The listing builds one solid part. Answer for the finished solid, in the listing's coordinates (mm). Give positions to 0.01 mm unless a question says otherwise; leave off trailing zeros. Loops run counter-clockwise (first coordinate to the right, second up) from the corner with the lowest first, then second, coordinate; pieces in that order, holes last. Notation, with made-up numbers: (78.25, 55) - (92.25, 55) arc R23 cw to (92.25, 90) - close; hole circle Ø10 at (1, 35.25). An arc over 180 degrees is marked (long way). Answer in a Markdown table with one row per item. Add a question column.
```python
from build123d import *

# Parameters (mm, degrees)
SKETCH1_R           = 4.25
SKETCH1_R_2         = 1.5
SKETCH1_W           = 40
SKETCH1_H           = 20
BOSS_EXTRUDE1_DEPTH = 6.1
SKETCH2_R           = 10.35
CUT_EXTRUDE1_DEPTH  = 2.55
SKETCH3_R           = 0.75
CUT_EXTRUDE3_DEPTH  = 3.55
CUT_EXTRUDE4_DEPTH  = 6.1


with BuildPart() as part:
    # Sketch1 → Boss-Extrude1 (new body)
    with BuildSketch(Plane(origin=(0, 0, 0), x_dir=(1, 0, 0), z_dir=(0, 1, 0))):
        with BuildLine():
            Line((150, 20), (159.5, 20))
            Line((159.5, 20), (166.5, 20))
            ThreePointArc((166.5, 20), (186.5, 0), (166.5, -20))
            Line((166.5, -20), (159.5, -20))
            Line((159.5, -20), (150, -20))
            Line((150, -20), (0, -20))
            ThreePointArc((0, -20), (-20, 0), (0, 20))
            Line((0, 20), (150, 20))
        make_face()
        with Locations(Location((0, 0, 0), (0, 0, 270))):
            Circle(SKETCH1_R, mode=Mode.SUBTRACT)
        with Locations(Location((165, 4.825, 0), (0, 0, 270))):
            Circle(SKETCH1_R_2, mode=Mode.SUBTRACT)
        with Locations(Location((165, -4.825, 0), (0, 0, 270))):
            Circle(SKETCH1_R_2, mode=Mode.SUBTRACT)
        with Locations(Location((114, 4.825, 0), (0, 0, 270))):
            Circle(SKETCH1_R_2, mode=Mode.SUBTRACT)
        with Locations(Location((114, -4.825, 0), (0, 0, 270))):
            Circle(SKETCH1_R_2, mode=Mode.SUBTRACT)
        with Locations((139.5, 0)):
            Rectangle(SKETCH1_W, SKETCH1_H, mode=Mode.SUBTRACT)
    extrude(amount=BOSS_EXTRUDE1_DEPTH)

    # Sketch2 → Cut-Extrude1 (cut)
    with BuildSketch(Plane(origin=(0, 6.1, 0), x_dir=(1, 0, 0), z_dir=(0, 1, 0))):
        with Locations(Location((0, 0, 0), (0, 0, 270))):
            Circle(SKETCH2_R)
    extrude(amount=-CUT_EXTRUDE1_DEPTH, mode=Mode.SUBTRACT)

    # Sketch3 → Cut-Extrude3 (cut)
    with BuildSketch(Plane(origin=(0, 3.55, 0), x_dir=(1, 0, 0), z_dir=(0, 1, 0))):
        with Locations(Location((-7.52500865, 2.715556079, 0), (0, 0, 270))):
            Circle(SKETCH3_R)
        with Locations(Location((7.52500865, -2.715556079, 0), (0, 0, 270))):
            Circle(SKETCH3_R)
        with Locations(Location((2.715556079, 7.52500865, 0), (0, 0, 270))):
            Circle(SKETCH3_R)
        with Locations(Location((-2.715556079, -7.52500865, 0), (0, 0, 270))):
            Circle(SKETCH3_R)
    extrude(amount=-CUT_EXTRUDE3_DEPTH, mode=Mode.SUBTRACT)

    # Sketch4 → Cut-Extrude4 (cut)
    with BuildSketch(Plane(origin=(0, 6.1, 0), x_dir=(1, 0, 0), z_dir=(0, 1, 0))):
        Polygon((32.320508076, 0), (27.990381057, 7.5), (19.330127019, 7.5), (15, 0), (19.330127019, -7.5), (27.990381057, -7.5), align=None)
        Polygon((57.320508076, 0), (52.990381057, 7.5), (44.330127019, 7.5), (40, 0), (44.330127019, -7.5), (52.990381057, -7.5), align=None)
        Polygon((82.320508076, 0), (77.990381057, 7.5), (69.330127019, 7.5), (65, 0), (69.330127019, -7.5), (77.990381057, -7.5), align=None)
        Polygon((107.320508076, 0), (102.990381057, 7.5), (94.330127019, 7.5), (90, 0), (94.330127019, -7.5), (102.990381057, -7.5), align=None)
        Polygon((30.490381057, 7.5), (42.037386441, 7.5), (39.150635095, 2.5), (33.377132403, 2.5), align=None)
        Polygon((64.150635095, 2.5), (67.037386441, 7.5), (55.490381057, 7.5), (58.377132403, 2.5), align=None)
        Polygon((89.150635095, 2.5), (92.037386441, 7.5), (80.490381057, 7.5), (83.377132403, 2.5), align=None)
        Polygon((30.490381057, -7.5), (42.037386441, -7.5), (39.150635095, -2.5), (33.377132403, -2.5), align=None)
        Polygon((55.490381057, -7.5), (67.037386441, -7.5), (64.150635095, -2.5), (58.377132403, -2.5), align=None)
        Polygon((80.490381057, -7.5), (92.037386441, -7.5), (89.150635095, -2.5), (83.377132403, -2.5), align=None)
    extrude(amount=-CUT_EXTRUDE4_DEPTH, mode=Mode.SUBTRACT)


solid = part.part
```
(1) Given pin 1 Ø3 at (y, z) = (4, -1.5) entering from -X; pin 2 Ø1.5 at (y, z) = (2.5, -7.5) entering from +X; pin 3 Ø1.5 at (y, z) = (1.5, 13.5) entering from -X, each flat-ended and moving along its own axis, determine where each tip first touches the part or whether it passes through.
(2) A cutting plane is placed at A-A on x = 125. Determine the outline of the cut face in (y, z), plus the area to 3 significant figures.
(3) A cutting plane is placed at C-C on z = 15.5. Determine the outline of the cut face in (x, y), plus the area to 3 significant figures.
(4) A cutting plane is placed at B-B on y = 1.5. Give the number of separate pieces and of enclosed holes in the cut face, plus the area to 3 significant figures.
(5) The mould has two halves that part along Z. Classify faces 1 (the face through (84, 3, 20)), 2 (the face through (61, 3, -7.5)): pulls with the +Z half, pulls with the -Z half, needs draft (parallel to the pull), parting line crosses it, or undercut.
(6) Find the intervals of material crossed by line 1 along Z through (x, y) = (114, 2) (3 decimals); line 2 along Z through (x, y) = (120.5, 1.75); line 3 along X through (y, z) = (5.5, 9.5), in increasing order. Write a range as [from, to].
Evaluation:
| question | item | result |
|---|---|---|
| 1 | pin 1 | stops at x = -20 |
| 1 | pin 2 | stops at x = 185.33 |
| 1 | pin 3 | stops at x = -15.41 |
| 2 | outline | (0, -20) - (6.1, -20) - (6.1, -10) - (0, -10) - close; (0, 10) - (6.1, 10) - (6.1, 20) - (0, 20) - close |
| 2 | area | 122 mm² |
| 3 | outline | (-12.64, 0) - (179.14, 0) - (179.14, 6.1) - (-12.64, 6.1) - close |
| 3 | area | 1,170 mm² |
| 4 | separate pieces | 1 |
| 4 | enclosed holes | 20 |
| 4 | area | 5,990 mm² |
| 5 | face 1 | pulls with the +Z half |
| 5 | face 2 | undercut |
| 6 | line 1 | z = [-20, -6.325], [-3.325, 3.325], [6.325, 20] |
| 6 | line 2 | z = [-20, -10], [10, 20] |
| 6 | line 3 | x = [-17.6, -4.11], [4.11, 119.5], [159.5, 184.1] |
